The drawing under review shows one solid part. Ordinate dimensions are in mm from its lowest x, y, z. A direction names the side the tool comes from. Give positions to 0.01 mm unless a question says otherwise; leave off trailing zeros. Order: outer loops, then holes, each group sorted by start corner. A loop starts at its lowest first (then second) coordinate and runs counter-clockwise, first axis right, second up. Notation, with made-up numbers: (85.25, 82) -> (90.25, 82) arc R7 cw to (90.25, 93) -> close; hole circle Ø2 at (-21.75, 71). An arc over 180 degrees is marked (long way). One line per item, written item: value.
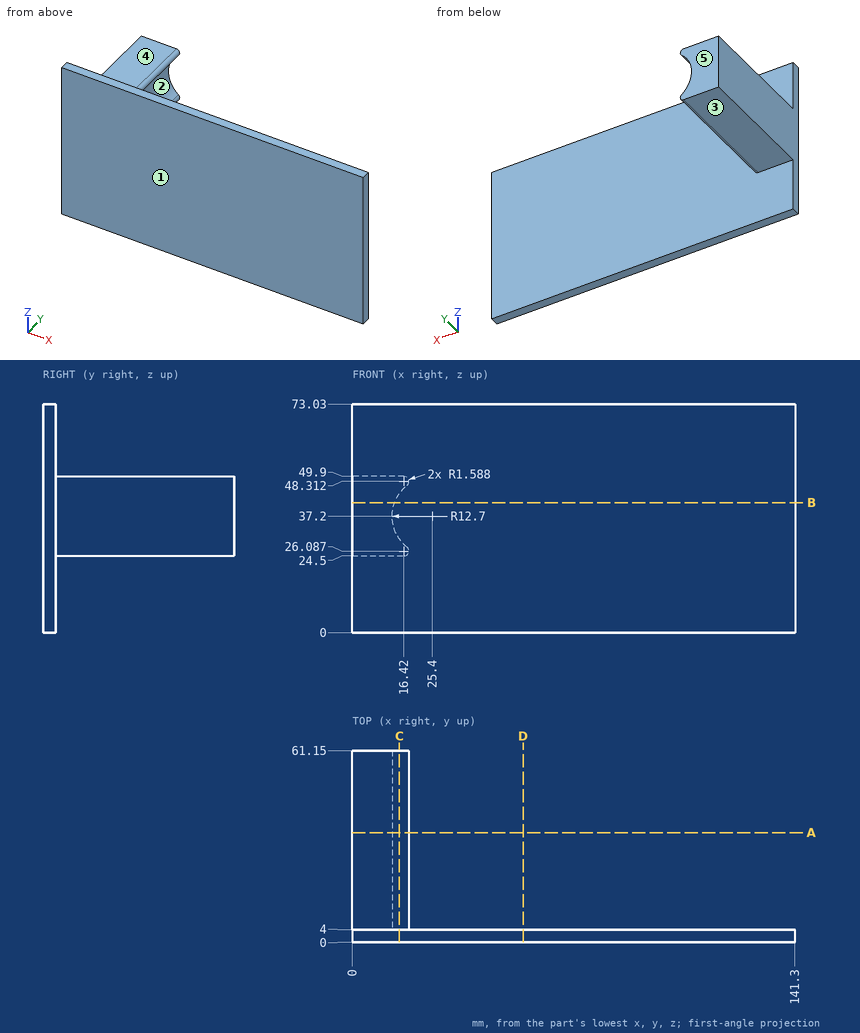
Item 1: Draft analysis for pull direction Z (two halves, no side actions). For the marked faces 1, 2 and 3, state which applies: pulls with the +Z half, pulls with the -Z half, needs draft (parallel to the pull), parting line crosses it, or undercut.
Returned:
face 1: needs draft
face 2: undercut
face 3: pulls with the -Z half
Item 2: Add section B-B on z = 41.5. Give the boundary of the cut face in (x, y), plus the area to 3 significant figures.
Returned:
outline: (0, 0) -> (141.3, 0) -> (141.3, 4) -> (13.45, 4) -> (13.45, 61.15) -> (0, 61.15) -> close
area: 1,330 mm²
Item 3: Clearance check with flat-ended pins moving along their axes: P1, Ø13, axis at x = 7.5, y = 26, coming from the -Z side; P2, Ø22, axis at x = 74.5, z = 53.5, coming from the +Y side; P3, Ø8, axis at x = 8.5, y = 44.5, coming from the +Z side. State where each tip first meets the part, or that it passes through.
Returned:
P1: z = 24.5
P2: y = 4
P3: z = 49.9
Item 4: Add section C-C on x = 15. Give the boundary of the cut face in (y, z).
Returned:
outline: (0, 0) -> (4, 0) -> (4, 24.5) -> (61.15, 24.5) -> (61.15, 29.91) -> (4, 29.91) -> (4, 44.49) -> (61.15, 44.49) -> (61.15, 49.9) -> (4, 49.9) -> (4, 73.03) -> (0, 73.03) -> close
Item 5: To check wall thickness, follow line 1 along Y through (x, z) = (95, 21); line 2 along Z through (x, y) = (8, 38); line 3 along X through (y, z) = (44.5, 26) (1 decimal). State the ranges of each line that lie inside material, in increasing order. Write a range as from..to.
Returned:
line 1: 0..4
line 2: 24.5..49.9
line 3: 0..18
Item 6: Machinability: for the marked faces 4 and 5, which of the approach directions +Z, -Z, +X, -X, +Y, -Y give a long, thin tool a straight path to every point of the face, cutting with its end or side? Answer none if there is none.
Returned:
face 4: +Z, +X, -X, +Y
face 5: +Z, -Z, +X, -X, +Y
Item 7: Add section A-A on y = 35. Give the boundary of the cut face in (x, z) (1 decimal).
Returned:
outline: (0, 24.5) -> (16.4, 24.5) arc R1.6 ccw to (17.4, 27.3) arc R12.7 cw to (17.4, 47.1) arc R1.6 ccw to (16.4, 49.9) -> (0, 49.9) -> close
Item 8: Add section D-D on x = 54.5. Give the boundary of the cut face in (y, z), plus the area to 3 significant figures.
Returned:
outline: (0, 0) -> (4, 0) -> (4, 73.03) -> (0, 73.03) -> close
area: 292 mm²
